Geometry: final body of the model. Coordinates: model frame, mm. A direction names the side the tool comes from. Give positions to 0.01 mm unless a question says otherwise; leave off trailing zeros. Write each loop counter-clockwise with the first axis right and the second up, starting at its lowest first coordinate (ties: lowest second). Pieces come first, ordered by that corner, then holes.
Q1. Cut plane D-D on y = 38.5. Return the cut outline in (x, z), plus the area to 3 significant figures.
Q2. Pin query (flat end, axial travel): pin 1 (1.5 mm diameter, centred on x = 46, z = 6, fed in from +Y); pin 2 (5 mm diameter, centred on y = 33, z = 4, fed in from -X). Return the tip coordinate at first contact, or that it passes through.
Q3. Cut plane B-B on y = 9. Return the cut outline in (x, z), plus the area to 3 significant figures.
Q4. Cut plane A-A on x = 22. Return the cut outline in (y, z).
Q5. Line query: L1, parallel to Y at x = 32, z = 2.5; L2, parallel to X at y = 6.5, z = 9; L3, parallel to Y at x = 9, z = 9.25. Output: solid intervals per line, ascending.
Q6. Draft query along X for faces 1 (the face through (0, 10, 5)), 2 (the face through (36, 16, 10)), 3 (the face through (28, 5.8, 5)). Return one class per face: pulls with the +X half, pulls with the -X half, needs draft (parallel to the pull), parting line crosses it, or undercut.
Q7. Cut plane C-C on z = 8.5. Return the cut outline in (x, y).
Q8. Reachability of faces 4 (the face through (36, 16, 0)), 5 (the face through (27, 12.2, 5)), 6 (the face through (52, 32, 5)) from +Z, -Z, +X, -X, +Y, -Y: full face, straight path, thin tool, end or side. Return the list, or none.
```python
from build123d import *

# Parameters (mm, degrees)
SKETCH_1_W          = 60
SKETCH_1_H          = 40
EXTRUDE_1_DEPTH     = 10
SKETCH_2_W          = 52
SKETCH_2_H          = 20
CUT_EXTRUDE_1_DEPTH = 73.801098893
FILLET_1_R          = 5
CUT_EXTRUDE_2_DEPTH = 73.801098893


with BuildPart() as part:
    # 草图1 → 凸台-拉伸1 (new body)
    with BuildSketch(Plane.XY):
        with Locations((30, 20)):
            Rectangle(SKETCH_1_W, SKETCH_1_H)
    extrude(amount=EXTRUDE_1_DEPTH)

    # 草图2 → 切除-拉伸1 (cut, through all)
    with BuildSketch(Plane.XY.offset(10)):
        with Locations((26, 30)):
            Rectangle(SKETCH_2_W, SKETCH_2_H)
    extrude(amount=-CUT_EXTRUDE_1_DEPTH, mode=Mode.SUBTRACT)

    # 圆角1
    fillet_1_edges = [part.edges().sort_by_distance(p)[0] for p in [
        (52, 20, 5),
    ]]
    fillet(fillet_1_edges, radius=FILLET_1_R)

    # 草图3 → 切除-拉伸2 (cut, through all)
    with BuildSketch(Plane.XY.offset(10)):
        with BuildLine():
            Line((10, 12.2), (45, 12.2))
            ThreePointArc((45, 12.2), (48.2, 9), (45, 5.8))
            Line((45, 5.8), (10, 5.8))
            ThreePointArc((10, 5.8), (6.8, 9), (10, 12.2))
        make_face()
    extrude(amount=-CUT_EXTRUDE_2_DEPTH, mode=Mode.SUBTRACT)


solid = part.part
```
Data:
1. outline: (52, 0) - (60, 0) - (60, 10) - (52, 10) - close
1. area: 80.0 mm2
2. pin 1: stops at y = 20
2. pin 2: stops at x = 52
3. outline: (0, 0) - (6.8, 0) - (6.8, 10) - (0, 10) - close; (48.2, 0) - (60, 0) - (60, 10) - (48.2, 10) - close
3. area: 186 mm2
4. outline: (0, 0) - (5.8, 0) - (5.8, 10) - (0, 10) - close; (12.2, 0) - (20, 0) - (20, 10) - (12.2, 10) - close
5. L1: y = 0 to 5.8, 12.2 to 20
5. L2: x = 0 to 8, 47 to 60
5. L3: y = 0 to 5.96, 12.04 to 20
6. face 1: pulls with the -X half
6. face 2: needs draft
6. face 3: undercut
7. outline: (0, 0) - (60, 0) - (60, 40) - (52, 40) - (52, 25) arc R5 cw to (47, 20) - (0, 20) - close; hole (10, 5.8) - (45, 5.8) arc R3.2 ccw to (45, 12.2) - (10, 12.2) arc R3.2 ccw to start
8. face 4: -Z, +X, -X, +Y, -Y
8. face 5: +Z, -Z
8. face 6: +Z, -Z, -X, +Y
